Model file for the job. Use its own axes, mm. A direction names the side the tool comes from. Round coordinates to 2 decimals unless told otherwise and drop trailing zeros. Order: outer loops, then holes, each group sorted by start corner. A loop starts at its lowest first (then second) coordinate and runs counter-clockwise, first axis right, second up. Notation, with made-up numbers: (-31, -15.75) -> (18, -15.75) arc R21 ccw to (18, -0.75) -> close; hole circle Ø1 at (-18, 6.5). An arc over 180 degrees is marked (long way). Use CSV: the item, a comma, the result in double quotes.
```python
from build123d import *

# Parameters (mm, degrees)
SKETCH_1_R          = 52
SKETCH_1_R_2        = 4.1
EXTRUDE_1_DEPTH     = 8
SKETCH_2_R          = 34
CUT_EXTRUDE_1_DEPTH = 2
FILLET_1_R          = 1
SKETCH_3_R          = 34
SKETCH_3_R_2        = 25
EXTRUDE_2_DEPTH     = 11.3
CHAMFER_1_SIZE      = 0.4
SKETCH_4_R          = 20
CUT_EXTRUDE_2_DEPTH = 10


with BuildPart() as part:
    # Эскиз1 → Бобышка-Вытянуть1 (new body)
    with BuildSketch(Plane.XY):
        Circle(SKETCH_1_R)
        with Locations((0, 44)):
            Circle(SKETCH_1_R_2, mode=Mode.SUBTRACT)
        with Locations((44, 0)):
            Circle(SKETCH_1_R_2, mode=Mode.SUBTRACT)
        with Locations((0, -44)):
            Circle(SKETCH_1_R_2, mode=Mode.SUBTRACT)
        with Locations((-44, 0)):
            Circle(SKETCH_1_R_2, mode=Mode.SUBTRACT)
    extrude(amount=EXTRUDE_1_DEPTH)

    # Эскиз2 → Вырез-Вытянуть1 (cut)
    with BuildSketch(Plane.XY.offset(8)):
        Circle(SKETCH_2_R)
    extrude(amount=-CUT_EXTRUDE_1_DEPTH, mode=Mode.SUBTRACT)

    # Скругление1
    fillet_1_edges = [part.edges().sort_by_distance(p)[0] for p in [
        (-34, 0, 6),
    ]]
    fillet(fillet_1_edges, radius=FILLET_1_R)

    # Эскиз3 → Бобышка-Вытянуть2 (add)
    with BuildSketch(Plane(origin=(0, 0, 0), x_dir=(-1, 0, 0), z_dir=(0, 0, -1))):
        with Locations(Location((0, 0, 0), (0, 0, 180))):
            Circle(SKETCH_3_R)
        Circle(SKETCH_3_R_2, mode=Mode.SUBTRACT)
    extrude(amount=EXTRUDE_2_DEPTH)

    # Фаска1
    chamfer_1_edges = [part.edges().sort_by_distance(p)[0] for p in [
        (25, 0, 0),
    ]]
    chamfer(chamfer_1_edges, length=CHAMFER_1_SIZE)

    # Эскиз4 → Вырез-Вытянуть2 (cut)
    with BuildSketch(Plane(origin=(0, 0, 0), x_dir=(-1, 0, 0), z_dir=(0, 0, -1))):
        Circle(SKETCH_4_R)
    extrude(amount=-CUT_EXTRUDE_2_DEPTH, mode=Mode.SUBTRACT)


solid = part.part
```
Q1. Cut at A-A (y = 0). State how many separate pieces and enclosed holes the cut face has, plus the area to 3 significant figures.
From the geometry:
separate pieces,"4"
enclosed holes,"0"
area,"529 mm²"
Q2. Pin check, flat tips, straight feed: pin 1 (3 mm diameter, centred on x = 11.5, z = 4, fed in from +Y); pin 2 (5 mm diameter, centred on y = -41.5, z = -0.5, fed in from +X); pin 3 (2 mm diameter, centred on y = 31.5, z = -6.5, fed in from -X) (3 decimals). Stop position of each tip, or through.
From the geometry:
pin 1,"stops at y = 51.03"
pin 2,"stops at x = 34.34"
pin 3,"stops at x = -15.025"
Q3. Which spindle directions (+Z, -Z, +X, -X, +Y, -Y) get a long thin tool onto all of the face, cutting with end or side? Do faces 1 (the cylindrical face through (18.28, 28.67, 7.51)), 2 (the flat face through (11, -34, 0)), 3 (the cylindrical face through (-41.265, -31.641, 3.944)). Say none if no direction does.
From the geometry:
face 1,"+Z"
face 2,"-Z"
face 3,"+Z, -Z"
Q4. Cut at B-B (z = 2). Give the cut face in (x, y).
From the geometry:
outline,"circle Ø104 at (0, 0); hole circle Ø8.2 at (-44, 0); hole circle Ø40 at (0, 0); hole circle Ø8.2 at (0, -44); hole circle Ø8.2 at (0, 44); hole circle Ø8.2 at (44, 0)"
Q5. Cut at C-C (x = -44). Give the cut face in (y, z), plus the area to 3 significant figures.
From the geometry:
outline,"(-27.71, 0) -> (-4.1, 0) -> (-4.1, 8) -> (-27.71, 8) -> close; (4.1, 0) -> (27.71, 0) -> (27.71, 8) -> (4.1, 8) -> close"
area,"378 mm²"
Q6. Probe line 1 along Y through (x, z) = (0, 3.7); line 2 along Z through (x, y) = (42, -21.5); line 3 along Z through (x, y) = (26.5, -7.5). List the from-to ranges inside material, lowest first.
From the geometry:
line 1,"y = -52 to -48.1, -39.9 to -20, 20 to 39.9, 48.1 to 52"
line 2,"z = 0 to 8"
line 3,"z = -11.3 to 6"
